CAD build for the part. Positions are in the model's coordinates, mm. Face numbers are marked on the shaded views. A direction names the side the tool comes from. Round coordinates to 2 decimals unless told otherwise and drop trailing zeros. Loops run counter-clockwise (first coordinate to the right, second up) from the corner with the lowest first, then second, coordinate; pieces in that order, holes last.
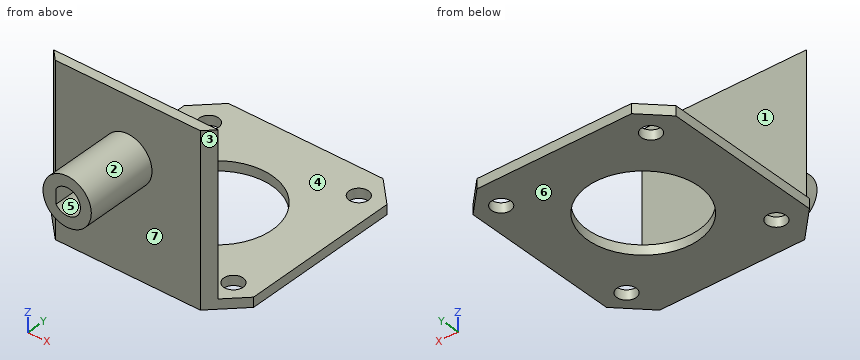
from build123d import *

# Parameters (mm, degrees)
SKETCH1_R           = 5
BOSS_EXTRUDE1_DEPTH = 15
CUT_EXTRUDE1_DEPTH  = 17.583123952
SKETCH3_W           = 42
SKETCH3_H           = 45
BOSS_EXTRUDE2_DEPTH = 2
SKETCH4_W           = 42
SKETCH4_H           = 2
BOSS_EXTRUDE3_DEPTH = 42
SKETCH6_R           = 11.5
CUT_EXTRUDE3_DEPTH  = 10
SKETCH7_W           = 42
SKETCH7_H           = 10
CUT_EXTRUDE4_DEPTH  = 10
SKETCH5_R           = 2
CUT_EXTRUDE5_DEPTH  = 10
CHAMFER1_SIZE       = 5
CHAMFER2_SIZE       = 6


with BuildPart() as part:
    # Sketch1 → Boss-Extrude1 (new body)
    with BuildSketch(Plane(origin=(0, 0, 0), x_dir=(1, 0, 0), z_dir=(0, 1, 0))):
        with Locations(Location((0, 0, 0), (0, 0, 270))):
            Circle(SKETCH1_R)
    extrude(amount=BOSS_EXTRUDE1_DEPTH)

    # Sketch2 → Cut-Extrude1 (cut, through all)
    with BuildSketch(Plane(origin=(0, 15, 0), x_dir=(1, 0, 0), z_dir=(0, 1, 0))):
        with BuildLine():
            Line((-2.28148439, 1.53535956), (-2.28148439, -1.53535956))
            ThreePointArc((-2.28148439, -1.53535956), (2.75, 0), (-2.28148439, 1.53535956))
        make_face()
    extrude(amount=-CUT_EXTRUDE1_DEPTH, mode=Mode.SUBTRACT)

    # Sketch3 → Boss-Extrude2 (add)
    with BuildSketch(Plane(origin=(0, 15, 0), x_dir=(1, 0, 0), z_dir=(0, 1, 0))):
        Rectangle(SKETCH3_W, SKETCH3_H)
    extrude(amount=BOSS_EXTRUDE2_DEPTH)

    # Sketch4 → Boss-Extrude3 (add)
    with BuildSketch(Plane(origin=(0, 17, 0), x_dir=(1, 0, 0), z_dir=(0, 1, 0))):
        with Locations((0, 21.5)):
            Rectangle(SKETCH4_W, SKETCH4_H)
    extrude(amount=BOSS_EXTRUDE3_DEPTH)

    # Sketch6 → Cut-Extrude3 (cut)
    with BuildSketch(Plane(origin=(0, 0, -22.5), x_dir=(-1, 0, 0), z_dir=(0, 0, -1))):
        with Locations((0, 37)):
            Circle(SKETCH6_R)
    extrude(amount=-CUT_EXTRUDE3_DEPTH, mode=Mode.SUBTRACT)

    # Sketch7 → Cut-Extrude4 (cut)
    with BuildSketch(Plane(origin=(0, 17, 0), x_dir=(1, 0, 0), z_dir=(0, 1, 0))):
        with Locations((0, -17.5)):
            Rectangle(SKETCH7_W, SKETCH7_H)
    extrude(amount=-CUT_EXTRUDE4_DEPTH, mode=Mode.SUBTRACT)

    # Sketch5 → Cut-Extrude5 (cut)
    with BuildSketch(Plane(origin=(0, 0, -22.5), x_dir=(-1, 0, 0), z_dir=(0, 0, -1))):
        with Locations((15, 53)):
            Circle(SKETCH5_R)
        with Locations((-16, 53)):
            Circle(SKETCH5_R)
        with Locations((15, 22)):
            Circle(SKETCH5_R)
        with Locations((-16, 22)):
            Circle(SKETCH5_R)
    extrude(amount=-CUT_EXTRUDE5_DEPTH, mode=Mode.SUBTRACT)

    # Chamfer1
    chamfer1_edges = [part.edges().sort_by_distance(p)[0] for p in [
        (-21, 59, -21.5),
        (21, 59, -21.5),
    ]]
    chamfer(chamfer1_edges, length=CHAMFER1_SIZE)

    # Chamfer2
    chamfer2_edges = [part.edges().sort_by_distance(p)[0] for p in [
        (21, 15, -5),
        (-21, 15, -5),
    ]]
    chamfer(chamfer2_edges, length=CHAMFER2_SIZE)


solid = part.part
Item 1: Cut at A-A (y = 53). List the corners of the cut face in (x, z).
Verdict:
outline: (-21, -22.5) - (-17, -22.5) - (-17, -20.5) - (-21, -20.5) - close; (-13, -22.5) - (14, -22.5) - (14, -20.5) - (-13, -20.5) - close; (18, -22.5) - (21, -22.5) - (21, -20.5) - (18, -20.5) - close
Item 2: Flat gauge pins, fed straight in: P1, Ø9, axis at x = -1, z = -10, coming from the -Y side; P2, Ø10, axis at x = 3.5, z = -1.5, coming from the +Y side; P3, Ø1.5, axis at y = 10, z = 0.5, coming from the +X side. Where does each tip first touch, or does it go through?
Verdict:
P1: stops at y = 15
P2: stops at y = 17
P3: stops at x = 5
Item 3: Cut at B-B (x = 0). List the corners of the cut face in (y, z), plus the area to 4 significant figures.
Verdict:
outline: (0, -5) - (15, -5) - (15, -22.5) - (25.5, -22.5) - (25.5, -20.5) - (17, -20.5) - (17, 12.5) - (15, 12.5) - (15, 5) - (0, 5) - (0, 2.75) - (15, 2.75) - (15, -2.75) - (0, -2.75) - close; (48.5, -22.5) - (59, -22.5) - (59, -20.5) - (48.5, -20.5) - close
area: 175.5 mm2
Item 4: Mould opens along Z. For the marked faces 4, 5, 6 and 7 say: released by +Z, released by -Z, zero draft, split by the parting line, or undercut.
Verdict:
face 4: released by +Z
face 5: undercut
face 6: released by -Z
face 7: zero draft
Item 5: 3-axis set-ups, long thin cutter, end or side, ignore diameter. For the marked faces 1, 2 and 3: which of +Z, -Z, +X, -X, +Y, -Y reach the whole face in a straight line?
Verdict:
face 1: +Z, +X, -X, +Y
face 2: -Y
face 3: +Z, -Z, +X, -Y
Item 6: Cut at D-D (z = 0). List the corners of the cut face in (x, y).
Verdict:
outline: (-17, 17) - (-15, 15) - (-5, 15) - (-5, 0) - (-2.28, 0) - (-2.28, 15) - (2.75, 15) - (2.75, 0) - (5, 0) - (5, 15) - (15, 15) - (17, 17) - close
Item 7: Cut at C-C (y = 37). List the corners of the cut face in (x, z).
Verdict:
outline: (-21, -22.5) - (-11.5, -22.5) - (-11.5, -20.5) - (-21, -20.5) - close; (11.5, -22.5) - (21, -22.5) - (21, -20.5) - (11.5, -20.5) - close
Item 8: Wall check: L1, parallel to Y at x = 16, z = -21.4; L2, parallel to Y at x = 0, z = -20.95; L3, parallel to Y at x = 11, z = 10. Give the ranges that are in metal, low to high.
Verdict:
L1: y = 16 to 20, 24 to 51, 55 to 59
L2: y = 15 to 25.5, 48.5 to 59
L3: y = 15 to 17
